Design review of the part built by this model. Coordinates are the model's own, in mm. A direction names the side the tool comes from. Give positions to 0.01 mm unless a question says otherwise; leave off trailing zeros. Write each loop counter-clockwise with the first axis right and the second up, starting at its lowest first coordinate (ties: lowest second). Pieces come first, ordered by that corner, then holes. Notation, with made-up numbers: (-23.75, 81) -> (12.25, 81) arc R9 ccw to (12.25, 86) -> close; hole circle Ø10 at (-7.75, -5). An arc over 180 degrees is marked (long way). Use CSV: the item, a comma, the result in double quotes.
```python
from build123d import *

# Parameters (mm, degrees)
SKETCH_1_W      = 15
SKETCH_1_H      = 15
EXTRUDE_1_DEPTH = 3
SKETCH_2_W      = 12.8
SKETCH_2_H      = 12.8
EXTRUDE_2_DEPTH = 10
CHAMFER_1_SIZE  = 1
FILLET_1_R      = 2
CHAMFER_2_SIZE  = 0.6


with BuildPart() as part:
    # 草图1 → 凸台-拉伸1 (new body)
    with BuildSketch(Plane(origin=(0, 0, 0), x_dir=(1, 0, 0), z_dir=(0, 1, 0))):
        Rectangle(SKETCH_1_W, SKETCH_1_H)
    extrude(amount=EXTRUDE_1_DEPTH)

    # 草图2 → 凸台-拉伸2 (add)
    with BuildSketch(Plane(origin=(0, 3, 0), x_dir=(1, 0, 0), z_dir=(0, 1, 0))):
        Rectangle(SKETCH_2_W, SKETCH_2_H)
    extrude(amount=EXTRUDE_2_DEPTH)

    # 倒角1
    chamfer_1_edges = [part.edges().sort_by_distance(p)[0] for p in [
        (0, 0, 7.5),
        (-7.5, 0, 0),
        (0, 0, -7.5),
        (7.5, 0, 0),
    ]]
    chamfer(chamfer_1_edges, length=CHAMFER_1_SIZE)

    # 圆角1
    fillet_1_edges = [part.edges().sort_by_distance(p)[0] for p in [
        (6.4, 8, 6.4),
        (6.4, 8, -6.4),
        (-6.4, 8, -6.4),
        (-6.4, 8, 6.4),
    ]]
    fillet(fillet_1_edges, radius=FILLET_1_R)

    # 倒角2
    chamfer_2_edges = [part.edges().sort_by_distance(p)[0] for p in [
        (0, 13, -6.4),
        (6.4, 13, 0),
        (-6.4, 13, 0),
        (0, 13, 6.4),
        (5.814213562, 13, 5.814213562),
        (-5.814213562, 13, 5.814213562),
        (-5.814213562, 13, -5.814213562),
        (5.814213562, 13, -5.814213562),
    ]]
    chamfer(chamfer_2_edges, length=CHAMFER_2_SIZE)


solid = part.part
```
(1) Take a section at C-C (z = -1). Write out the cut boundary in (x, y).
Established:
outline,"(-7.5, 1) -> (-6.5, 0) -> (6.5, 0) -> (7.5, 1) -> (7.5, 3) -> (6.4, 3) -> (6.4, 12.4) -> (5.8, 13) -> (-5.8, 13) -> (-6.4, 12.4) -> (-6.4, 3) -> (-7.5, 3) -> close"
(2) Take a section at A-A (x = 3). Write out the cut boundary in (y, z).
Established:
outline,"(0, -6.5) -> (1, -7.5) -> (3, -7.5) -> (3, -6.4) -> (12.4, -6.4) -> (13, -5.8) -> (13, 5.8) -> (12.4, 6.4) -> (3, 6.4) -> (3, 7.5) -> (1, 7.5) -> (0, 6.5) -> close"
(3) Take a section at B-B (y = 5.5). Write out the cut boundary in (x, z).
Established:
outline,"(-6.4, -4.4) arc R2 ccw to (-4.4, -6.4) -> (4.4, -6.4) arc R2 ccw to (6.4, -4.4) -> (6.4, 4.4) arc R2 ccw to (4.4, 6.4) -> (-4.4, 6.4) arc R2 ccw to (-6.4, 4.4) -> close"
(4) Tool access review of faces 1 (the face through (0, 8, 6.4)), 2 (the face through (0, 8, -6.4)), 3 (the face through (-5.8, 7.77, -5.83)), 4 (the face through (6.4, 8, 0)), 5 (the face through (-5.8, 7.77, 5.83)): name each direction out of +Z, -Z, +X, -X, +Y, -Y from which nothing blocks a thin tool from reaching the whole face with its end or side.
Established:
face 1,"+Z, +X, -X, +Y"
face 2,"-Z, +X, -X, +Y"
face 3,"-Z, -X, +Y"
face 4,"+Z, -Z, +X, +Y"
face 5,"+Z, -X, +Y"
(5) Clearance check with flat-ended pins moving along their axes: pin 1 (1 mm diameter, centred on x = 1, y = 6, fed in from +Z); pin 2 (2.5 mm diameter, centred on x = 1.5, y = 8.5, fed in from -Z); pin 3 (4.5 mm diameter, centred on y = 6.5, z = 0, fed in from -X). State where each tip first meets the part, or that it passes through.
Established:
pin 1,"stops at z = 6.4"
pin 2,"stops at z = -6.4"
pin 3,"stops at x = -6.4"
(6) For line 1 along Z through (x, y) = (1.5, 6.25); line 2 along X through (y, z) = (10, 5), list the stretches that pass through material, from the lowest coordinate up. Write a range as [from, to].
Established:
line 1,"z = [-6.4, 6.4]"
line 2,"x = [-6.31, 6.31]"
